from build123d import *

# Parameters (mm, degrees)
SKETCH1_R           = 4.7625
SKETCH1_R_2         = 2.032
BOSS_EXTRUDE1_DEPTH = 1.5875
BOSS_EXTRUDE2_START = -1.5875
SKETCH2_R           = 2.032
BOSS_EXTRUDE2_DEPTH = 1.5875


with BuildPart() as part:
    # Sketch1 → Boss-Extrude1 (new body)
    with BuildSketch(Plane(origin=(0, 0, 0), x_dir=(0, 0, -1), z_dir=(1, 0, 0))):
        with BuildLine():
            Line((-3.367596045, 22.417596045), (-22.417596045, 3.367596045))
            ThreePointArc((-22.417596045, 3.367596045), (-23.8125, 0), (-22.417596045, -3.367596045))
            Line((-22.417596045, -3.367596045), (-3.367596045, -22.417596045))
            ThreePointArc((-3.367596045, -22.417596045), (1.253587833, -23.64455371), (4.611270797, -20.240625))
            Line((4.611270797, -20.240625), (9.222541593, -2.38125))
            ThreePointArc((9.222541593, -2.38125), (9.525, 0), (9.222541593, 2.38125))
            Line((9.222541593, 2.38125), (4.611270797, 20.240625))
            ThreePointArc((4.611270797, 20.240625), (1.253587833, 23.64455371), (-3.367596045, 22.417596045))
        make_face()
        Circle(SKETCH1_R, mode=Mode.SUBTRACT)
        with Locations((0, 19.05)):
            Circle(SKETCH1_R_2, mode=Mode.SUBTRACT)
        with Locations((-19.05, 0)):
            Circle(SKETCH1_R_2, mode=Mode.SUBTRACT)
        with Locations((0, -19.05)):
            Circle(SKETCH1_R_2, mode=Mode.SUBTRACT)
    extrude(amount=BOSS_EXTRUDE1_DEPTH)

    # Sketch2 → Boss-Extrude2 (add)
    with BuildSketch(Plane(origin=(1.5875, 0, 0), x_dir=(0, 0, -1), z_dir=(1, 0, 0)).offset(BOSS_EXTRUDE2_START)):
        with BuildLine():
            Line((-3.115398581, -22.652179609), (-32.484148581, 2.747820391))
            ThreePointArc((-32.484148581, 2.747820391), (-33.699944523, 4.369555541), (-34.13125, 6.35))
            Line((-34.13125, 6.35), (-34.13125, 19.05))
            ThreePointArc((-34.13125, 19.05), (-32.736346045, 22.417596045), (-29.36875, 23.8125))
            Line((-29.36875, 23.8125), (0, 23.8125))
            ThreePointArc((0, 23.8125), (-1.822529847, 23.449976274), (-3.367596045, 22.417596045))
            Line((-3.367596045, 22.417596045), (-22.417596045, 3.367596045))
            ThreePointArc((-22.417596045, 3.367596045), (-23.8125, 0), (-22.417596045, -3.367596045))
            Line((-22.417596045, -3.367596045), (-3.367596045, -22.417596045))
            ThreePointArc((-3.367596045, -22.417596045), (-3.243618688, -22.537168487), (-3.115398581, -22.652179609))
        make_face()
        with Locations((-29.36875, 6.35)):
            Circle(SKETCH2_R, mode=Mode.SUBTRACT)
        with Locations((-29.36875, 19.05)):
            Circle(SKETCH2_R, mode=Mode.SUBTRACT)
    extrude(amount=BOSS_EXTRUDE2_DEPTH)


solid = part.part
The listing builds one solid part. Answer for the finished solid, in the listing's coordinates (mm). Round coordinates to 2 decimals unless told otherwise and drop trailing zeros. Loops run counter-clockwise (first coordinate to the right, second up) from the corner with the lowest first, then second, coordinate; pieces in that order, holes last. Notation, with made-up numbers: M 16,39 L 37,39 A30 ccw 37,64 Z; hole C -32,-8 d11. An arc over 180 degrees is marked long. Write each question's results on one line, items separated by ' | '. Start each with the question number.
1) Straight lines are drawn through the part: probe 1 along Y at (x, z) = (0.95, 0); probe 2 along Z at (x, y) = (0.7, 18); probe 3 along Y at (x, z) = (0.95, 30). For each, find the intervals that lie inside material, in ascending order.
2) Find section D-D on z = 20.5. Write down the section's boundary in (x, y), plus the area to 3 significant figures.
3) Find section B-B on y = 0. Write down the section's boundary in (x, z) (1 decimal), plus the area to 3 significant figures.
4) Determine the mould class of faces 1 (the cylindrical face through (0.783, 22.38, 32.773)), 2 (the cylindrical face through (0.783, -0.034, -9.525)), 3 (the cylindrical face through (0.783, -17.337, -1.092)) for opening direction Z: pulls with the +Z half, pulls with the -Z half, needs draft (parallel to the pull), parting line crosses it, or undercut.
5) Find section A-A on x = 1.05. Count the separate pieces of the cut face and the enclosed holes in it, plus the area to 3 significant figures.
6) Find section C-C on z = -1.5. Write down the section's boundary in (x, y), plus the area to 3 significant figures.
7) Each of these flat-tipped pins is pushed along its axis until it touches: pin 1 (3 mm diameter, centred on y = -3.5, z = 17.5, fed in from -X); pin 2 (2.5 mm diameter, centred on y = 6.35, z = 29.37, fed in from +X). Where does it stop, or does it pass through?
Final values:
1) probe 1: -23.81 to -21.08, -17.02 to -4.76, 4.76 to 17.02, 21.08 to 23.81 | probe 2: -5.19 to -1.74, 1.74 to 27.63, 31.11 to 34.13 | probe 3: 0.6 to 4.42, 8.28 to 17.12, 20.98 to 23.77
2) outline: M 0,-7.62 L 1.59,-7.62 L 1.59,-1.42 L 0,-1.42 Z; M 0,1.42 L 1.59,1.42 L 1.59,23.81 L 0,23.81 Z | area: 45.4 mm²
3) outline: M 0,-9.5 L 1.6,-9.5 L 1.6,-4.8 L 0,-4.8 Z; M 0,4.8 L 1.6,4.8 L 1.6,17 L 0,17 Z; M 0,21.1 L 1.6,21.1 L 1.6,29.3 L 0,29.3 Z | area: 40.1 mm²
4) face 1: pulls with the +Z half | face 2: pulls with the -Z half | face 3: undercut
5) separate pieces: 1 | enclosed holes: 6 | area: 1,350 mm²
6) outline: M 0,-23.57 L 1.59,-23.57 L 1.59,-20.42 L 0,-20.42 Z; M 0,-17.68 L 1.59,-17.68 L 1.59,-4.52 L 0,-4.52 Z; M 0,4.52 L 1.59,4.52 L 1.59,17.68 L 0,17.68 Z; M 0,20.42 L 1.59,20.42 L 1.59,23.57 L 0,23.57 Z | area: 51.8 mm²
7) pin 1: x = 0 | pin 2: through
